Verification items for the finished model (mm, model axes). Round coordinates to 2 decimals unless told otherwise and drop trailing zeros. Order: outer loops, then holes, each group sorted by start corner. A loop starts at its lowest first (then second) coordinate and runs counter-clockwise, first axis right, second up. Notation, with made-up numbers: (72, 57.5) -> (107, 57.5) arc R13 cw to (107, 75.5) -> close; hole circle Ø7 at (53.5, -8.75). An arc over 180 degrees is marked (long way). Put each result on its own line as item: value.
Autodesk Inventor part; units mm, degrees
ref_plane "YZ Plane" through (0, 0, 0) normal (1, 0, 0) x (0, 1, 0)
ref_plane "XZ Plane" through (0, 0, 0) normal (0, 1, 0) x (-1, 0, 0)
ref_plane "XY Plane" through (0, 0, 0) normal (0, 0, 1) x (1, 0, 0)
sketch "Boceto1" plane through (0, 0, 0) normal (0, 1, 0) x (-1, 0, 0)
  line L0 (0, 0) -> (-75, 0)
  line L1 (-75, 0) -> (-75, -80)
  line L2 (-75, -80) -> (0, -80)
  line L3 (0, -80) -> (0, 0)
  dimension "d0" = 80
  dimension "d1" = 75
extrude "Extrusión1" add sketch "Boceto1" along normal blind 6
sketch "Boceto2" plane through (0, 6, 0) normal (0, 1, 0) x (1, 0, 0)
  line L0 (0, 0) -> (75, 0)
  line L1 (25, 0) -> (25, 8)
  line L2 (25, 8) -> (7.5, 8)
  line L3 (7.5, 8) -> (7.5, 27.5)
  line L4 (7.5, 27.5) -> (0, 27.5)
  line L5 (0, 27.5) -> (0, 40)
  line L6 (25, 0) -> (50, 0)
  line L7 (50, 0) -> (50, 8)
  line L8 (50, 8) -> (75, 8)
  line L9 (75, 0) -> (75, 80)
  line L10 (-21.9373, 40) -> (100.0778, 40)
  line L11 (25, 0) -> (50, 0)
  line L12 (25, 80) -> (25, 72)
  line L13 (25, 72) -> (7.5, 72)
  line L14 (7.5, 72) -> (7.5, 52.5)
  line L15 (7.5, 52.5) -> (0, 52.5)
  line L16 (0, 52.5) -> (0, 40)
  line L17 (50, 80) -> (50, 72)
  line L18 (50, 72) -> (75, 72)
  line L19 (25, 80) -> (50, 80)
  line L20 (75, 80) -> (0, 80)
  line L21 (0, 80) -> (0, 0)
  dimension "d4" = 12.5
  dimension "d7" = 8
  dimension "d8" = 25
  dimension "d9" = 25
  dimension "d10" = 12.5
  dimension "d11" = 27.5
  dimension "d12" = 27.5
  dimension "d13" = 8
  dimension "d14" = 8
  dimension "d15" = 8
  dimension "d16" = 7.5
  dimension "d17" = 25
  dimension "d18" = 25
  dimension "d19" = 25
  dimension "d20" = 25
extrude "Extrusión2" cut sketch "Boceto2" against normal through all contours L21 L4 L3 L2 L1 L0 | L7 L8 L9 L0 | L21 L20 L12 L13 L14 L15 | L18 L17 L20 L9
sketch "Boceto3" plane through (0, 6, 0) normal (0, 1, 0) x (1, 0, 0)
  circle A0 centre (3.75, 40) radius 1.5
  circle A1 centre (37.5, 76) radius 1.5
  circle A2 centre (37.5, 4) radius 1.5
  line L0 (7.5, 52.5) -> (0, 52.5)
  line L1 (0, 52.5) -> (0, 27.5)
  line L2 (50, 80) -> (25, 80)
  line L3 (25, 0) -> (50, 0)
  line L4 (50, 0) -> (50, 8)
  line L5 (50, 72) -> (50, 80)
  point P0 (0, 0)
  dimension "d23" = 3
  dimension "d24" = 12.5
  dimension "d25" = 3.75
  dimension "d26" = 4
  dimension "d27" = 4
  dimension "d28" = 12.5
  dimension "d29" = 12.5
extrude "Extrusión3" cut sketch "Boceto3" against normal through all
sketch "Boceto4" plane through (0, 6, 0) normal (0, 1, 0) x (1, 0, 0)
  circle A0 centre (3.75, 40) radius 1.5
  circle A1 centre (3.75, 40) radius 3.1
  circle A2 centre (37.5, 4) radius 1.5
  circle A3 centre (37.5, 4) radius 3.1
  circle A4 centre (37.5, 76) radius 1.5
  circle A5 centre (37.5, 76) radius 3.1
  point P0 (0, 0)
  dimension "d32" = 6.2
extrude "Extrusión4" cut sketch "Boceto4" against normal blind 2.5 contours A0 | A1 | A2 | A3 | A5
sketch "Boceto5" plane through (0, 6, 0) normal (0, 1, 0) x (1, 0, 0)
  line L0 (0, 52.5) -> (0, 27.5)
  line L1 (7.5, 52.5) -> (0, 52.5)
  line L2 (0, 52.5) -> (7.5, 52.5)
  line L3 (7.5, 52.5) -> (7.5, 52.3)
  line L4 (7.5, 52.3) -> (0, 52.3)
  line L5 (0, 52.3) -> (0, 52.5)
  line L6 (25, 80) -> (25, 72)
  line L7 (25, 80) -> (25.2, 80)
  line L8 (25.2, 80) -> (25.2, 71.85)
  line L9 (25.2, 71.85) -> (25, 71.85)
  line L10 (25, 71.85) -> (25, 80)
  line L11 (7.5, 72) -> (25, 72)
  line L12 (25, 72) -> (25, 71.85)
  line L13 (25, 71.85) -> (7.5, 71.85)
  line L14 (7.5, 71.85) -> (7.5, 72)
  line L15 (7.5, 52.3) -> (7.65, 52.3)
  line L16 (7.65, 52.3) -> (7.65, 72)
  line L17 (7.65, 72) -> (7.5, 72)
  line L18 (7.5, 72) -> (7.5, 52.3)
  line L19 (50, 80) -> (25, 80)
  line L20 (50, 80) -> (49.8, 80)
  line L21 (49.8, 80) -> (49.8, 71.85)
  line L22 (49.8, 71.85) -> (50, 71.85)
  line L23 (50, 71.85) -> (50, 80)
  line L24 (50, 71.85) -> (75, 71.85)
  line L25 (75, 71.85) -> (75, 72)
  line L26 (75, 72) -> (50, 72)
  line L27 (50, 72) -> (50, 71.85)
  line L28 (50, 8) -> (75, 8)
  line L29 (75, 8) -> (74.8, 8)
  line L30 (74.8, 8) -> (74.8, 72)
  line L31 (74.8, 72) -> (75, 72)
  line L32 (75, 72) -> (75, 8)
  line L33 (-2.8758, 40) -> (82.3038, 40)
  line L34 (7.5, 27.5) -> (0, 27.5)
  line L35 (0, 27.5) -> (7.5, 27.5)
  line L36 (7.5, 27.5) -> (7.5, 27.7)
  line L37 (7.5, 27.7) -> (0, 27.7)
  line L38 (0, 27.7) -> (0, 27.5)
  line L39 (25, 0) -> (25, 8)
  line L40 (25, 0) -> (25.2, 0)
  line L41 (25.2, 0) -> (25.2, 8.15)
  line L42 (25.2, 8.15) -> (25, 8.15)
  line L43 (25, 8.15) -> (25, 0)
  line L44 (7.5, 8) -> (25, 8)
  line L45 (25, 8) -> (25, 8.15)
  line L46 (25, 8.15) -> (7.5, 8.15)
  line L47 (7.5, 8.15) -> (7.5, 8)
  line L48 (7.5, 27.7) -> (7.65, 27.7)
  line L49 (7.65, 27.7) -> (7.65, 8)
  line L50 (7.65, 8) -> (7.5, 8)
  line L51 (7.5, 8) -> (7.5, 27.7)
  line L52 (50, 0) -> (49.8, 0)
  line L53 (49.8, 0) -> (49.8, 8.15)
  line L54 (49.8, 8.15) -> (50, 8.15)
  line L55 (50, 8.15) -> (50, 0)
  line L56 (50, 8.15) -> (75, 8.15)
  line L57 (75, 8.15) -> (75, 8)
  line L58 (75, 8) -> (50, 8)
  line L59 (50, 8) -> (50, 8.15)
  point P0 (0, 0)
  point P1 (7.5, 8.15)
  point P2 (7.65, 8.15)
  point P3 (0, 27.7)
  point P4 (74.8, 71.85)
  point P5 (74.8, 8.15)
  point P6 (0, 52.3)
  point P7 (7.65, 71.85)
  point P8 (7.5, 71.85)
  dimension "d35" = 0.2
  dimension "d36" = 0.15
  dimension "d37" = 0.2
  dimension "d38" = 0.15
  dimension "d39" = 0.2
  dimension "d40" = 0.15
  dimension "d41" = 0.2
extrude "Extrusión5" cut sketch "Boceto5" against normal blind 6 contours L1 L3 L4 L0 | L37 L36 L34 L0 | L18 L13 L16 L15 L3 | L14 L11 L16 L13 | L33 L32 L56 L30 | L30 L24 L32 L33 | L16 L11 L10 L13 | L48 L49 L46 L51 L36 | L56 L32 L28 L30 | L30 L28 L55 L56 | L30 L26 L25 L24 | L24 L23 L26 L30 | L10 L6 L7 L8 L9 | L55 L52 L53 L54 | L22 L21 L19 L23 | L46 L49 L44 L47 | L46 L43 L44 L49 | L42 L41 L40 L39 L43
sketch "Boceto6" plane through (0, 6, 0) normal (0, 1, 0) x (1, 0, 0)
  point P0 (0, 0)
sketch "Boceto7" plane through (0, 6, 0) normal (0, 1, 0) x (1, 0, 0)
  line L0 (13.5, 17.5) -> (68.5, 17.5)
  line L1 (68.5, 17.5) -> (68.5, 62.5)
  line L2 (68.5, 62.5) -> (13.5, 62.5)
  line L3 (13.5, 62.5) -> (13.5, 17.5)
  line L4 (0, 52.3) -> (0, 27.7)
  line L5 (49.8, 80) -> (25.2, 80)
  line L6 (13.5, 17.5) -> (16, 17.5)
  line L7 (16, 17.5) -> (16, 62.5)
  line L8 (16, 62.5) -> (13.5, 62.5)
  line L9 (13.5, 62.5) -> (13.5, 17.5)
  line L10 (18.5, 17.5) -> (18.5, 62.5)
  line L11 (21, 17.5) -> (21, 62.5)
  line L12 (23.5, 17.5) -> (23.5, 62.5)
  line L13 (26, 17.5) -> (26, 62.5)
  line L14 (28.5, 17.5) -> (28.5, 62.5)
  line L15 (31, 17.5) -> (31, 62.5)
  line L16 (33.5, 17.5) -> (33.5, 62.5)
  line L17 (36, 17.5) -> (36, 62.5)
  line L18 (38.5, 17.5) -> (38.5, 62.5)
  line L19 (41, 17.5) -> (41, 62.5)
  line L20 (43.5, 17.5) -> (43.5, 62.5)
  line L21 (46, 17.5) -> (46, 62.5)
  line L22 (48.5, 17.5) -> (48.5, 62.5)
  line L23 (51, 17.5) -> (51, 62.5)
  line L24 (53.5, 17.5) -> (53.5, 62.5)
  line L25 (56, 17.5) -> (56, 62.5)
  line L26 (58.5, 17.5) -> (58.5, 62.5)
  line L27 (61, 17.5) -> (61, 62.5)
  line L28 (63.5, 17.5) -> (63.5, 62.5)
  line L29 (66, 17.5) -> (66, 62.5)
  point P0 (0, 0)
  point P1 (0, 40)
  point P2 (37.5, 80)
  dimension "d44" = 45
  dimension "d45" = 55
  dimension "d46" = 22.5
  dimension "d47" = 31
  dimension "d48" = 2.5
  dimension "d51" = 2.5
extrude "Extrusión6" cut sketch "Boceto7" against normal blind 6 contours L7 L2 L10 L0 | L11 L2 L12 L0 | L13 L2 L14 L0 | L15 L2 L16 L0 | L17 L2 L18 L0 | L19 L2 L20 L0 | L21 L2 L22 L0 | L23 L2 L24 L0 | L25 L2 L26 L0 | L27 L2 L28 L0 | L29 L2 L1 L0
fillet "Empalme1" radius 0.7 22 edges at (66, 6, -40) (63.5, 6, -40) (61, 6, -40) (58.5, 6, -40) (56, 6, -40) (53.5, 6, -40) (51, 6, -40) (48.5, 6, -40) (46, 6, -40) (43.5, 6, -40) (41, 6, -40) (38.5, 6, -40) (68.5, 6, -40) (36, 6, -40) (33.5, 6, -40) (31, 6, -40) (28.5, 6, -40) (26, 6, -40) (23.5, 6, -40) (21, 6, -40) (18.5, 6, -40) (16, 6, -40)
properties part number "Tapa - Caja para Electrónica"
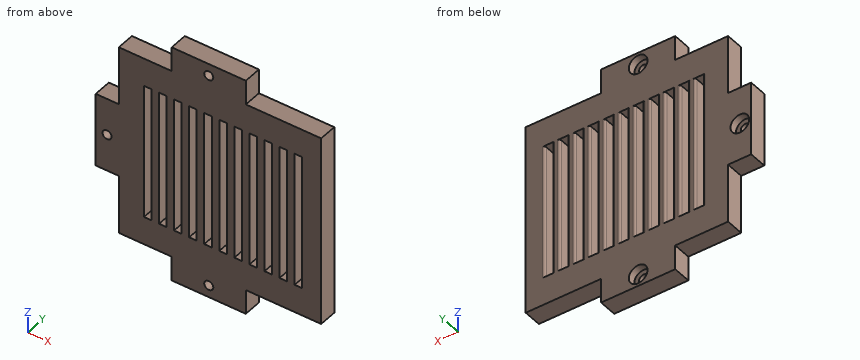
Item 1: Sectioned sample at D-D, the plane z = -22.5. Give the number of separate pieces and of enclosed holes in the cut face, then the cut area to 3 significant figures.
Geometry check:
separate pieces: 12
enclosed holes: 0
area: 236 mm2
Item 2: Sectioned sample at C-C, the plane x = 37.5. Record the boundary of the cut face in (y, z), then the cut area to 3 significant figures.
Geometry check:
outline: (0, -80) -> (6, -80) -> (6, -79.1) -> (3.5, -79.1) -> (3.5, -77.5) -> (0, -77.5) -> close; (0, -74.5) -> (3.5, -74.5) -> (3.5, -72.9) -> (6, -72.9) -> (6, -62.5) -> (0, -62.5) -> close; (0, -17.5) -> (6, -17.5) -> (6, -7.1) -> (3.5, -7.1) -> (3.5, -5.5) -> (0, -5.5) -> close; (0, -2.5) -> (3.5, -2.5) -> (3.5, -0.9) -> (6, -0.9) -> (6, 0) -> (0, 0) -> close
area: 158 mm2
Item 3: Material ranges on line 1 along Z through (x, y) = (37.5, 0.95); line 2 along Z through (x, y) = (37.5, 4.6); line 3 along X through (y, z) = (4.15, -4), recorded low to high.
Geometry check:
line 1: -80 to -77.5, -74.5 to -62.5, -17.5 to -5.5, -2.5 to 0
line 2: -80 to -79.1, -72.9 to -62.5, -17.5 to -7.1, -0.9 to 0
line 3: 25.2 to 34.4, 40.6 to 49.8
Item 4: Sectioned sample at A-A, the plane x = 3.75. Record the boundary of the cut face in (y, z), then the cut area to 3 significant figures.
Geometry check:
outline: (0, -52.3) -> (6, -52.3) -> (6, -43.1) -> (3.5, -43.1) -> (3.5, -41.5) -> (0, -41.5) -> close; (0, -38.5) -> (3.5, -38.5) -> (3.5, -36.9) -> (6, -36.9) -> (6, -27.7) -> (0, -27.7) -> close
area: 122 mm2
Item 5: Sectioned sample at B-B, the plane z = -4. Record the boundary of the cut face in (x, y), then the cut area to 3 significant figures.
Geometry check:
outline: (25.2, 0) -> (36, 0) -> (36, 3.5) -> (34.4, 3.5) -> (34.4, 6) -> (25.2, 6) -> close; (39, 0) -> (49.8, 0) -> (49.8, 6) -> (40.6, 6) -> (40.6, 3.5) -> (39, 3.5) -> close
area: 122 mm2
Item 6: Depth check by flat-ended pin: pin 1 Ø5 at (x, z) = (3.75, -40) entering from +Y; pin 2 Ø3 at (x, z) = (43.5, -37) entering from -Y; pin 3 Ø1 at (y, z) = (0.5, -58) entering from -X; pin 4 Ø3 at (x, y) = (67, 3.5) entering from +Z. Enter the tip coordinate at first touch or a pass-through.
Geometry check:
pin 1: y = 3.5
pin 2: y = 0
pin 3: x = 7.65
pin 4: z = -8.15
